from build123d import *

# Parameters (mm, degrees)
F0_W     = 50
F0_H     = 20
F1_DEPTH = 381
F2_R     = 25.220427
F3_DEPTH = 50
F5_DEPTH = 12.7


with BuildPart() as f1:
    # F0 (on Front) → F1 (new body, symmetric)
    with BuildSketch(Plane.XZ):
        Rectangle(F0_W, F0_H)
    extrude(amount=F1_DEPTH, both=True)

    # F2 (on face) → F3 (join)
    with BuildSketch(Plane(origin=(0, 0, -10), x_dir=(1, 0, 0), z_dir=(0, 0, -1))):
        with Locations((0, -356)):
            Circle(F2_R)
    extrude(amount=F3_DEPTH)

    # F4 (on face) → F5 (join)
    with BuildSketch(Plane.XY.offset(10)):
        Polygon((-152.4, -76.2), (-152.4, -381), (0, -381), (152.4, -381), (152.4, -76.2), align=None)
    extrude(amount=F5_DEPTH)


solid = f1.part
Part model, mm, in its own coordinate system. A direction names the side the tool comes from. Give positions to 0.01 mm unless a question says otherwise; leave off trailing zeros. Loops run counter-clockwise (first coordinate to the right, second up) from the corner with the lowest first, then second, coordinate; pieces in that order, holes last. Notation, with made-up numbers: (-34, -5.75) -> (5, -5.75) arc R26 ccw to (5, 33.25) -> close; hole circle Ø6 at (30.25, 88.25). An arc over 180 degrees is marked (long way). Write each question's results on one line, items separated by ' | '. Start each with the question number.
Q1. Wall check: L1, parallel to Y at x = 2, z = -11; L2, parallel to Z at x = 44, y = -114; L3, parallel to X at y = 316.5, z = -5. Give the ranges that are in metal, low to high.
Q2. Pin check, flat tips, straight feed: P1, Ø4, axis at y = 134, z = 0.5, coming from the -X side; P2, Ø22, axis at x = -4, z = -1, coming from the +Y side; P3, Ø6, axis at y = -48, z = 4.5, coming from the +X side. Stop position of each tip, or through.
Q3. Band-saw the part on A-A on y = -152. List the corners of the cut face in (x, z), plus the area to 3 significant figures.
Q4. Which spindle directions (+Z, -Z, +X, -X, +Y, -Y) get a long thin tool onto all of the face, cutting with end or side? Do faces 1 (the face through (88, -226, 10)), 2 (the face through (0, 149, 10)), 3 (the face through (-5.47, 380.62, -34.65)), 4 (the face through (-90, -226, 10)). Say none if no direction does.
Q5. Band-saw the part on C-C on x = -86.5. List the corners of the cut face in (y, z).
Q6. Band-saw the part on B-B on z = -0.5. List the corners of the cut face in (x, y), plus the area to 3 significant figures.
Q7. Band-saw the part on D-D on z = -38. List the corners of the cut face in (x, y).
Results are:
1) L1: y = 330.86 to 381.14 | L2: z = 10 to 22.7 | L3: x = -25 to 25
2) P1: stops at x = -25 | P2: stops at y = 381.22 | P3: stops at x = 25
3) outline: (-152.4, 10) -> (-25, 10) -> (-25, -10) -> (25, -10) -> (25, 10) -> (152.4, 10) -> (152.4, 22.7) -> (-152.4, 22.7) -> close | area: 4,870 mm²
4) face 1: -Z, +X, +Y, -Y | face 2: +Z, +X, -X, +Y | face 3: -Z | face 4: -Z, -X, +Y, -Y
5) outline: (-381, 10) -> (-76.2, 10) -> (-76.2, 22.7) -> (-381, 22.7) -> close
6) outline: (-25, -381) -> (25, -381) -> (25, 381) -> (-25, 381) -> close | area: 38,100 mm²
7) outline: circle Ø50.44 at (0, 356)
